Autodesk Inventor part; units mm, degrees
ref_plane "YZ Plane" through (0, 0, 0) normal (1, 0, 0) x (0, 1, 0)
ref_plane "XZ Plane" through (0, 0, 0) normal (0, 1, 0) x (-1, 0, 0)
ref_plane "XY Plane" through (0, 0, 0) normal (0, 0, 1) x (1, 0, 0)
sketch "Sketch1" plane through (0, 0, 0) normal (0, 0, 1) x (1, 0, 0)
  line L0 (-2.9393, 4) -> (2.9393, 4)
  line L1 (4, 2.9393) -> (4, -2.9393)
  line L2 (2.9393, -4) -> (-2.9393, -4)
  line L3 (-4, -2.9393) -> (-4, 2.9393)
  line L4 (0, 0) -> (4, -4) construction
  line L5 (-0.5303, -0.5303) -> (-4, -4) construction
  line L6 (5.0607, 4) -> (10, 4) construction
  line L7 (8.2426, 7.182) -> (8.2426, 3.2426)
  line L8 (8.2426, 3.2426) -> (10.2426, 3.2426)
  line L9 (10.2426, 3.2426) -> (10.2426, 10.2426)
  line L10 (10.2426, 10.2426) -> (3.2426, 10.2426)
  line L11 (3.2426, 10.2426) -> (3.2426, 8.2426)
  line L12 (3.2426, 8.2426) -> (7.182, 8.2426)
  line L13 (2.9393, 4) -> (7.182, 8.2426)
  line L14 (4, 2.9393) -> (8.2426, 7.182)
  line L15 (-8.2426, 7.182) -> (-8.2426, 3.2426)
  line L16 (-8.2426, 3.2426) -> (-10.2426, 3.2426)
  line L17 (-10.2426, 3.2426) -> (-10.2426, 10.2426)
  line L18 (-10.2426, 10.2426) -> (-3.2426, 10.2426)
  line L19 (-3.2426, 10.2426) -> (-3.2426, 8.2426)
  line L20 (-3.2426, 8.2426) -> (-7.182, 8.2426)
  line L21 (-2.9393, 4) -> (-7.182, 8.2426)
  line L22 (-4, 2.9393) -> (-8.2426, 7.182)
  line L23 (-2.9393, -4) -> (2.9393, -4)
  line L24 (4, -2.9393) -> (4, 2.9393)
  line L25 (-4, 2.9393) -> (-4, -2.9393)
  line L26 (-4, -4) -> (0, 0) construction
  line L27 (5.0607, -4) -> (10, -4) construction
  line L28 (8.2426, -7.182) -> (8.2426, -3.2426)
  line L29 (8.2426, -3.2426) -> (10.2426, -3.2426)
  line L30 (10.2426, -3.2426) -> (10.2426, -10.2426)
  line L31 (10.2426, -10.2426) -> (3.2426, -10.2426)
  line L32 (3.2426, -10.2426) -> (3.2426, -8.2426)
  line L33 (3.2426, -8.2426) -> (7.182, -8.2426)
  line L34 (2.9393, -4) -> (7.182, -8.2426)
  line L35 (4, -2.9393) -> (8.2426, -7.182)
  line L36 (-3.2426, -10.2426) -> (-3.2426, -8.2426)
  line L37 (-2.9393, -4) -> (-7.182, -8.2426)
  line L38 (-8.2426, -7.182) -> (-8.2426, -3.2426)
  line L39 (-3.2426, -8.2426) -> (-7.182, -8.2426)
  line L40 (-4, -2.9393) -> (-8.2426, -7.182)
  line L41 (-10.2426, -3.2426) -> (-10.2426, -10.2426)
  line L42 (-10.2426, -10.2426) -> (-3.2426, -10.2426)
  line L43 (-8.2426, -3.2426) -> (-10.2426, -3.2426)
  point P0 (0, 0)
  point P1 (-4, 4)
  point P2 (-4, 4)
  dimension "d0" = 8
extrude "Extrusion1" add sketch "Sketch1" along normal mid plane 300
move faces "이동3" translate (0, 0, 80) faces at (-1.3333, 0.9798, 150)
move faces "이동4" translate (0, 0, -41) faces at (-1.3333, 1.6869, 230)
move faces "이동5" translate (0, 0, -169) faces at (-1.3333, 1.6869, 189)
properties part number "Beam 380 mm"
Design review of the part built by this model. Coordinates are the model's own, in mm. A direction names the side the tool comes from. Give positions to 0.01 mm unless a question says otherwise; leave off trailing zeros. Order: outer loops, then holes, each group sorted by start corner. A loop starts at its lowest first (then second) coordinate and runs counter-clockwise, first axis right, second up. Notation, with made-up numbers: M -31.75,-16.75 L 11.25,-16.75 A18 ccw 11.25,-0.75 Z; hole C -6.5,28.5 d4. An arc over 180 degrees is marked long. One line per question, with ' | ' between items. Start each with the question number.
Q1. The part is to be moulded in two halves that separate along Y. For faces 3 (the face through (-7, 10.243, -66)), 4 (the face through (-5.03, 6.09, -66.19)), 5 (the face through (-5, 8.243, -66)), 6 (the face through (0, -4, -66)), say which applies: +Y half, -Y half, draft (parallel to the pull), parting line (faces both ways), or undercut.
Q2. Machinability: for faces 1 (the face through (0, 0, -150)), 2 (the face through (4, 0, -66)), which of the approach directions +Z, -Z, +X, -X, +Y, -Y give a long, thin tool a straight path to every point of the face, cutting with its end or side? Answer none if there is none.
Q3. For pin 1 Ø4.5 at (y, z) = (0.5, -26.5) entering from -X; pin 2 Ø3 at (x, z) = (-0.5, -31.5) entering from +Y; pin 3 Ø1.8 at (x, z) = (0, -41.5) entering from -Y, all flat-tipped, find the tip position at first contact; note any pin that passes through.
Q4. For L1, parallel to Y at x = -6.5, z = 13; L2, parallel to Y at x = -9, z = 4.5; L3, parallel to Y at x = -6.75, z = -64.5, list the stretches that pass through material, from the lowest coordinate up. Write a range as [from, to].
Q5. We need section A-A (x = -1.5). Write out the cut boundary in (y, z), plus the area to 3 significant figures.
Returned:
1) face 3: +Y half | face 4: undercut | face 5: undercut | face 6: -Y half
2) face 1: -Z, +X, -X, +Y, -Y | face 2: +Z, -Z, +X
3) pin 1: x = -4 | pin 2: y = 4 | pin 3: y = -4
4) L1: [-10.24, -8.24], [-7.56, -5.44], [5.44, 7.56], [8.24, 10.24] | L2: [-10.24, -3.24], [3.24, 10.24] | L3: [-10.24, -8.24], [-7.81, -5.69], [5.69, 7.81], [8.24, 10.24]
5) outline: M -4,-150 L 4,-150 L 4,20 L -4,20 Z | area: 1,360 mm2
